Autodesk Inventor part; units mm, degrees
ref_plane "YZ Plane" through (0, 0, 0) normal (1, 0, 0) x (0, 1, 0)
ref_plane "XZ Plane" through (0, 0, 0) normal (0, 1, 0) x (-1, 0, 0)
ref_plane "XY Plane" through (0, 0, 0) normal (0, 0, 1) x (1, 0, 0)
sketch "Sketch1" plane through (0, 0, 0) normal (0, 0, 1) x (1, 0, 0)
  line L0 (0.0065, 132.461) -> (0.0065, 0) construction
  line L1 (-17.4935, 132.461) -> (-17.4935, 0)
  line L2 (17.5065, 0) -> (17.5065, 132.461)
  arc A0 (17.5065, 132.461) -> (-17.4935, 132.461) centre (0.0065, 132.461) ccw
  arc A1 (-17.4935, 0) -> (17.5065, 0) centre (0.0065, 0) ccw
  circle A2 centre (0.0065, 0) radius 11.1
  circle A3 centre (0.0065, 131.961) radius 7.5
  line L3 (4.0065, 131.961) -> (4.0065, 109.961)
  line L4 (4.0065, 109.961) -> (-3.9935, 109.961)
  line L5 (-3.9935, 109.961) -> (-3.9935, 131.961)
  line L6 (-3.9935, 131.961) -> (4.0065, 131.961)
  line L7 (0.0065, 101.721) -> (0.0065, -30.5)
  line L8 (0.0065, 131.961) -> (5.7519, 127.1401)
  line L9 (0.0065, 131.961) -> (0.0065, 124.461) construction
  arc A4 (5.7519, 127.1401) -> (4.0065, 122.4546) centre (13.9526, 121.4175) ccw
  line L10 (0.0065, 131.961) -> (-5.7388, 127.1401)
  arc A5 (-3.9935, 122.4546) -> (-5.7388, 127.1401) centre (-13.9395, 121.4175) ccw
  line L11 (0.0065, 132.461) -> (0.0065, 108.461) construction
  line L12 (4.0065, 132.461) -> (4.0065, 108.461)
  line L13 (-3.9935, 108.461) -> (-3.9935, 132.461)
  arc A6 (4.0065, 132.461) -> (-3.9935, 132.461) centre (0.0065, 132.461) ccw
  arc A7 (-3.9935, 108.461) -> (4.0065, 108.461) centre (0.0065, 108.461) ccw
  point P0 (0.0065, 131.961)
  point P1 (-3.9935, 122.4546)
  point P2 (-5.7388, 127.1401)
  point P3 (0.0065, 120.461)
  point P4 (-3.9935, 109.961)
  point P5 (4.0065, 109.961)
  dimension "d38" = 15
  dimension "d19" = 35
  dimension "d20" = 22.2
  dimension "d39" = 22
  dimension "d40" = 8
  dimension "d41" = 4
  dimension "d42" = 4
  dimension "d43" = 50
  dimension "d44" = 5
  dimension "d45" = 10
  dimension "d50" = 24
  dimension "d59" = 132.461
extrude "Extrusion1" add sketch "Sketch1" along normal mid plane 6
sketch "Sketch6" plane through (0, 0, 3) normal (0, 0, 1) x (1, 0, 0)
  arc A0 (-17.4935, 0) -> (17.5065, 0) centre (0.0065, 0) ccw
  line L0 (17.5065, 0) -> (17.5065, 132.461)
  arc A1 (17.5065, 132.461) -> (-17.4935, 132.461) centre (0.0065, 132.461) ccw
  line L1 (-17.4935, 132.461) -> (-17.4935, 0)
  arc A2 (-3.9935, 108.461) -> (4.0065, 108.461) centre (0.0065, 108.461) ccw
  line L2 (-3.9935, 108.461) -> (-3.9935, 122.4546)
  arc A3 (-3.9935, 122.4546) -> (-5.7388, 127.1401) centre (-13.9395, 121.4175) ccw
  arc A4 (5.7519, 127.1401) -> (-5.7388, 127.1401) centre (0.0065, 131.961) ccw
  arc A5 (5.7519, 127.1401) -> (4.0065, 122.4546) centre (13.9526, 121.4175) ccw
  line L3 (4.0065, 122.4546) -> (4.0065, 108.461)
  circle A6 centre (0.0065, 0) radius 11.1
  point P0 (0, 0)
extrude "Extrusion4" add sketch "Sketch6" along normal blind 2 contours L1 A1 L0 A0 | L2 A3 A4 A5 L3 A2
sketch "Sketch7" plane through (0, 0, 5) normal (0, 0, 1) x (1, 0, 0)
  line L0 (0, 244.3) -> (0, -244.3)
  line L1 (17.5065, 0) -> (17.5065, 132.461)
  arc A0 (17.5065, 132.461) -> (-17.4935, 132.461) centre (0.0065, 132.461) ccw
  line L2 (-17.4935, 132.461) -> (-17.4935, 0)
  arc A1 (-17.4935, 0) -> (17.5065, 0) centre (0.0065, 0) ccw
  circle A2 centre (0.0065, 0) radius 11.1
  circle A3 centre (0.0065, 0) radius 4.1
  point P0 (0, 0)
  point P1 (0, 11.1)
  point P2 (0, -11.1)
  point P3 (0, -17.5)
  point P4 (0, 149.961)
  dimension "d53" = 8.2
extrude "Extrusion5" add sketch "Sketch7" along normal blind 10 contours A0 L1 A1 L0 A2 | L0 A2 A1 L2 A0 | A2 L0 A3 | L0 A3 A2
sketch "Sketch9" plane through (0, 0, -3) normal (0, 0, -1) x (-1, 0, 0)
  line L0 (-4.0065, 122.4546) -> (-4.0065, 108.461)
  arc A0 (-4.0065, 108.461) -> (3.9935, 108.461) centre (-0.0065, 108.461) ccw
  line L1 (3.9935, 108.461) -> (3.9935, 122.4546)
  arc A1 (5.7388, 127.1401) -> (3.9935, 122.4546) centre (13.9395, 121.4175) ccw
  arc A2 (5.7388, 127.1401) -> (-5.7519, 127.1401) centre (-0.0065, 131.961) ccw
  arc A3 (-4.0065, 122.4546) -> (-5.7519, 127.1401) centre (-13.9526, 121.4175) ccw
  line L2 (4.1935, 122.4442) -> (4.1935, 108.461)
  arc A4 (-4.2065, 108.461) -> (4.1935, 108.461) centre (-0.0065, 108.461) ccw
  line L3 (-4.2065, 108.461) -> (-4.2065, 122.4442)
  arc A5 (-4.2065, 122.4442) -> (-5.9109, 127.0184) centre (-13.9526, 121.4175) ccw
  arc A6 (5.8978, 127.0184) -> (-5.9109, 127.0184) centre (-0.0065, 131.961) ccw
  arc A7 (5.8978, 127.0184) -> (4.1935, 122.4442) centre (13.9395, 121.4175) ccw
  point P0 (0, 0)
  dimension "d60" = 0.2
extrude "Extrusion7" cut sketch "Sketch9" against normal up to surface (6 mm away)
sketch "Sketch11" plane through (0, 0, 15) normal (0, 0, 1) x (1, 0, 0)
  line L0 (10.9002, -1.9232) -> (15.7624, 25.6515)
  line L1 (10.9002, -1.9232) -> (38.9002, -1.9232) construction
  circle A0 centre (-0.0065, 0) radius 11.075
  circle A1 centre (-0.0065, 0) radius 12
  line L2 (16.7472, 25.4778) -> (12.092, -0.9232)
  line L3 (12.8079, 26.1724) -> (7.325, -4.9232)
  circle A2 centre (-0.0065, 0) radius 13
  circle A3 centre (-0.0065, 0) radius 10
  line L4 (12.8079, 26.1724) -> (16.7472, 25.4778)
  point P0 (0, 0)
  point P1 (0, 0)
  point P2 (9.7149, 8.631)
  point P3 (12.7213, 2.6461)
  dimension "d74" = 28
  dimension "d75" = 80
  dimension "d76" = 24
  dimension "d77" = 1
  dimension "d78" = 3
  dimension "d80" = 2
extrude "Extrusion10" cut sketch "Sketch11" against normal blind 8 contours A2 L3 L4 L0 | L0 L4 L2 A2
sketch "Sketch13" plane through (0, 0, -3) normal (0, 0, -1) x (-1, 0, 0)
  line L0 (0, 101.0671) -> (0, 16.0671) construction
  line L1 (-10, 91.0671) -> (-10, 26.0671)
  line L2 (10, 26.0671) -> (10, 91.0671)
  arc A0 (10, 91.0671) -> (-10, 91.0671) centre (0, 91.0671) ccw
  arc A1 (-10, 26.0671) -> (10, 26.0671) centre (0, 26.0671) ccw
  line L3 (10, 26.0671) -> (10, 58.9004)
  line L4 (-10, 91.0671) -> (-10, 58.2338)
  line L5 (-10, 26.0671) -> (10, 58.9004)
  line L6 (10, 58.9004) -> (-10, 58.2338)
  line L7 (-10, 58.2338) -> (10, 91.0671)
  line L8 (33.0369, 58.1675) -> (-10, 56.7329)
  line L9 (32.9369, 61.1658) -> (-10.05, 59.7329)
  line L10 (-8.719, 57.4534) -> (11.281, 90.2868)
  line L11 (-11.281, 59.0141) -> (9.7071, 93.4696)
  line L12 (-9.7071, 23.6646) -> (11.281, 58.1201)
  line L13 (-11.281, 26.8474) -> (8.719, 59.6808)
  point P0 (0, 0)
  point P1 (0, 58.5671)
  point P2 (39.2224, 129.4846)
  point P3 (-10, 61.1171)
  point P4 (-10, 107.6003)
  point P5 (7.2741, 57.3087)
  point P6 (-10, 28.9505)
  point P7 (10, 56.017)
  point P8 (10, 60.4013)
  point P9 (-7.2741, 59.8255)
  point P10 (10, 88.1837)
  dimension "d97" = 20
  dimension "d98" = 65
  dimension "d99" = 32.8333
  dimension "d100" = 32.8333
  dimension "d101" = 1.5
  dimension "d102" = 1.5
  dimension "d103" = 1.5
  dimension "d104" = 1.5
  dimension "d105" = 1.5
  dimension "d106" = 1.5
extrude "Extrusion12" cut sketch "Sketch13" against normal up to next contours L8 L13 L1 | L1 A0 L11 | L10 L2 L9 | L12 L2 A1
fillet "Fillet2" radius 2 10 edges at (-9.7071, 93.4696, 6) (-10, 88.1837, 6) (10, 28.9505, 6) (10, 61.1171, 6) (-7.2741, 57.3087, 6) (-10, 56.017, 6) (9.7071, 23.6646, 6) (-10, 60.4013, 6) (7.2741, 59.8255, 6) (10, 56.7329, 6)
move or copy body "Move1" bodies to move or copy 1 copy no translate (0, -131.75, 0)
move or copy body "Move2" bodies to move or copy 1 copy no translate (0, 0, -6)
properties part number "EslabonRodillaCadera" material "PLA"
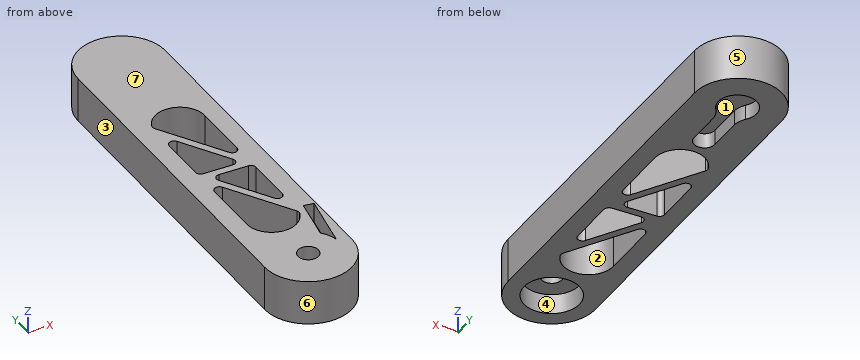
The listing builds one solid part. Answer for the finished solid, in the listing's coordinates (mm). Face numbers are marked on the shaded views. A direction names the side the tool comes from. Coordinates: 2 decimals unless noted, no trailing zeros. Loops run counter-clockwise (first coordinate to the right, second up) from the corner with the lowest first, then second, coordinate; pieces in that order, holes last.
1) Find the intervals of material crossed by L1, parallel to X at y = -131.75, z = 5; L2, parallel to X at y = 0, z = -8; L3, parallel to Y at x = -2, z = 6.75, in increasing order.
2) Determine the mould class of the marked faces 4, 5, 6 and 7 for opening direction Y: pulls with the +Y half, pulls with the -Y half, needs draft (parallel to the pull), parting line crosses it, or undercut.
3) A tool of negligible diameter and unlimited length cuts with its end or side. For the marked faces 1, 2 and 3, from which of +Z, -Z, +X, -X, +Y, -Y can it reach the whole face along a straight path? Write none if from no direction.
4) Find section A-A on x = -13. Write down the section's boundary in (y, z).
5) Flat-ended cylindrical pins translate along their axes: pin 1 Ø8 at (x, z) = (-12, 3.5) entering from +Y; pin 2 Ø6 at (x, z) = (8, -3) entering from -Y; pin 3 Ø6.5 at (x, y) = (4.5, -133.5) entering from -Z. Find the tip coordinate at first contact, or state that the pin passes through.
Values:
1. L1: x = -17.49 to -4.09, 4.11 to 17.51
1. L2: x = -17.49 to -7.69, 7.7 to 17.51
1. L3: y = -149.13 to -135.33, -128.17 to -115.48, -88.87 to -83.1, -74.62 to -71.62, -56.7 to -50.93, -30.88 to 18.1
2. face 4: undercut
2. face 5: pulls with the +Y half
2. face 6: pulls with the -Y half
2. face 7: needs draft
3. face 1: -Z
3. face 2: +Z, -Z
3. face 3: +Z, -Z, -X, +Y, -Y
4. outline: (-143.46, -9) - (12.42, -9) - (12.42, 9) - (-143.46, 9) - close
5. pin 1: stops at y = 16.27
5. pin 2: stops at y = -148.52
5. pin 3: stops at z = -1
